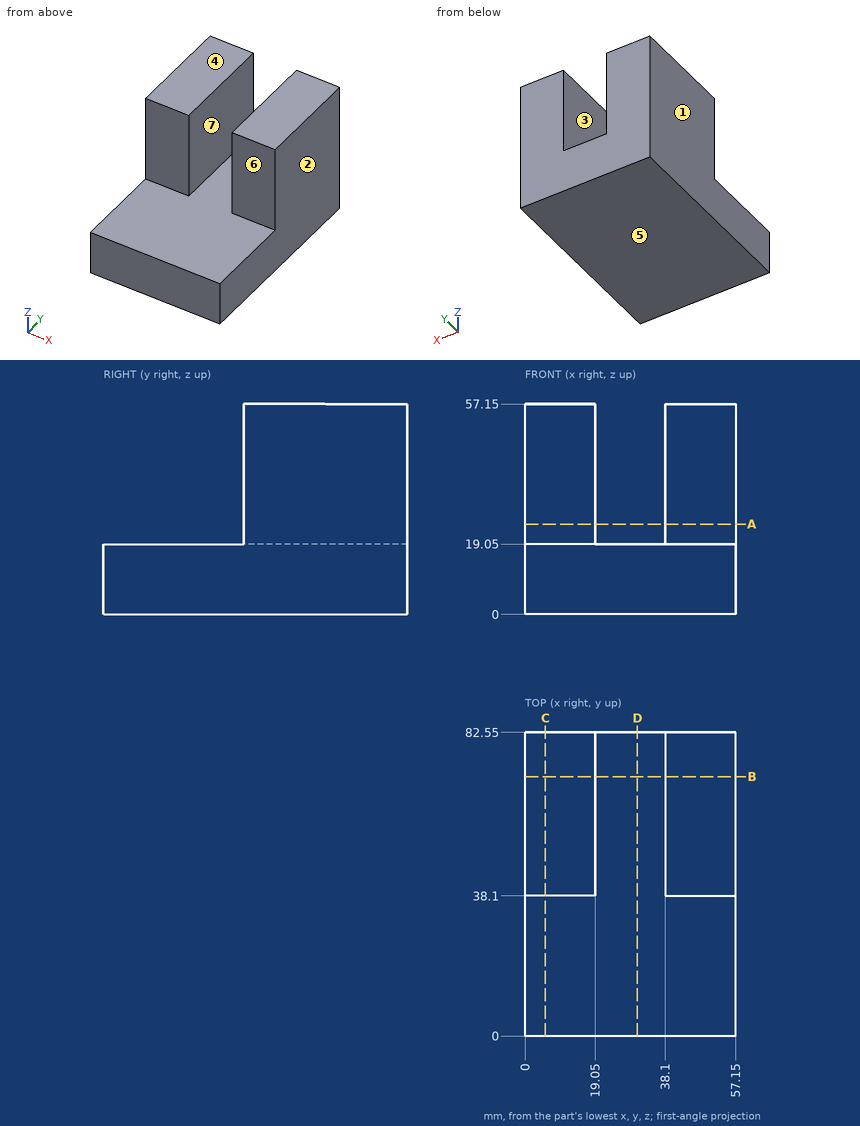
Here's the drawing with two shaded views (mm, measured from the low corner). I have some questions. A direction names the side the tool comes from. Coordinates: 2 decimals unless noted, no trailing zeros. Loops run counter-clockwise (first coordinate to the right, second up) from the corner with the lowest first, then second, coordinate; pieces in that order, holes last. Notation, with made-up numbers: (69.25, -2.5) - (108.25, -2.5) arc R12 cw to (108.25, 15.5) - close; hole circle Ø4 at (70.5, 34). An arc over 180 degrees is marked (long way). Answer as CSV lines item,"result". Start each with the question number.
1) Thinking about a two-plate mould opening in X: for the marked faces 1, 2, 3 and 4, which applies, pulls with the +X half, pulls with the -X half, needs draft (parallel to the pull), parting line crosses it, or undercut?
2) Suppose I cut it at D-D (x = 30.5). Please give me the cut outline in (y, z), plus the area to 3 significant figures.
3) I need wall thicknesses on line 1 (X direction, y = 58.5, z = 51.5); line 2 (Z direction, x = 30.5, y = 76); line 3 (Y direction, x = 4.5, z = 50). Which ranges of each line are inside material? Lowest first, please. Write a range as from..to.
4) Suppose I cut it at C-C (x = 5.5). Please give me the cut outline in (y, z), plus the area to 3 significant figures.
5) Suppose I cut it at B-B (y = 70.5). Please give me the cut outline in (x, z), plus the area to 3 significant figures.
6) For pin 1 (5.5 mm diameter, centred on x = 46.5, z = 39, fed in from -Y); pin 2 (10 mm diameter, centred on x = 21.5, y = 25, fed in from +Z); pin 3 (1 mm diameter, centred on x = 32.5, y = 30.5, fed in from -Z), each with a flat end and sliding along its axis, tell me the tip position at first contact or that it passes through.
7) Which directions (+Z, -Z, +X, -X, +Y, -Y) give clear straight access to the entire face, cutting with the end or side of a thin tool? Please do the marked faces 5, 6 and 7.
8) Suppose I cut it at A-A (z = 24.5). Please give me the cut outline in (x, y), plus the area to 3 significant figures.
Check result:
1,face 1,"pulls with the -X half"
1,face 2,"pulls with the +X half"
1,face 3,"undercut"
1,face 4,"needs draft"
2,outline,"(0, 0) - (82.55, 0) - (82.55, 19.05) - (0, 19.05) - close"
2,area,"1,570 mm²"
3,line 1,"x = 0..19.05, 38.1..57.15"
3,line 2,"z = 0..19.05"
3,line 3,"y = 38.1..82.55"
4,outline,"(0, 0) - (82.55, 0) - (82.55, 57.15) - (38.1, 57.15) - (38.1, 19.05) - (0, 19.05) - close"
4,area,"3,270 mm²"
5,outline,"(0, 0) - (57.15, 0) - (57.15, 57.15) - (38.1, 57.15) - (38.1, 19.05) - (19.05, 19.05) - (19.05, 57.15) - (0, 57.15) - close"
5,area,"2,540 mm²"
6,pin 1,"stops at y = 38.1"
6,pin 2,"stops at z = 19.05"
6,pin 3,"stops at z = 0"
7,face 5,"-Z, +X, -X, +Y, -Y"
7,face 6,"+Z, +X, -X, -Y"
7,face 7,"+Z, +Y, -Y"
8,outline,"(0, 38.1) - (19.05, 38.1) - (19.05, 82.55) - (0, 82.55) - close; (38.1, 38.1) - (57.15, 38.1) - (57.15, 82.55) - (38.1, 82.55) - close"
8,area,"1,690 mm²"
